The drawing under review shows one solid part. Ordinate dimensions are in mm from its lowest x, y, z. Round coordinates to 2 decimals unless told otherwise and drop trailing zeros. Order: outer loops, then holes, each group sorted by start corner. A loop starts at its lowest first (then second) coordinate and runs counter-clockwise, first axis right, second up. Notation, with made-up numbers: M 72,7.5 L 126,7.5 A17 ccw 126,39.5 Z; hole C 89,84.25 d9. An arc over 180 degrees is marked long. Answer as a JSON object with one key per item and string values. Group by question number.
1) Consider section B-B, the plane x = 72. Write out the cut boundary in (y, z).
2) Insertion check: pin 1 Ø4 at (x, y) = (59.2, 207.89) entering from -Z. The pin has a flat end and moves straight along its axis. Give the tip position at first contact, or say it passes through.
3) Consider section C-C, the plane z = 1.1. Count the separate pieces of the cut face and the enclosed holes in it, then the cut area to 3 significant figures.
4) Consider section A-A, the plane y = 88.5. Write out the cut boundary in (x, z).
5) To check wall thickness, follow line 1 (X direction, y = 257.89, z = 1.65); line 2 (Y direction, x = 138.5, z = 3.4); line 3 (Y direction, x = 173.8, z = 2.5). State the ranges of each line that lie inside material, in increasing order.
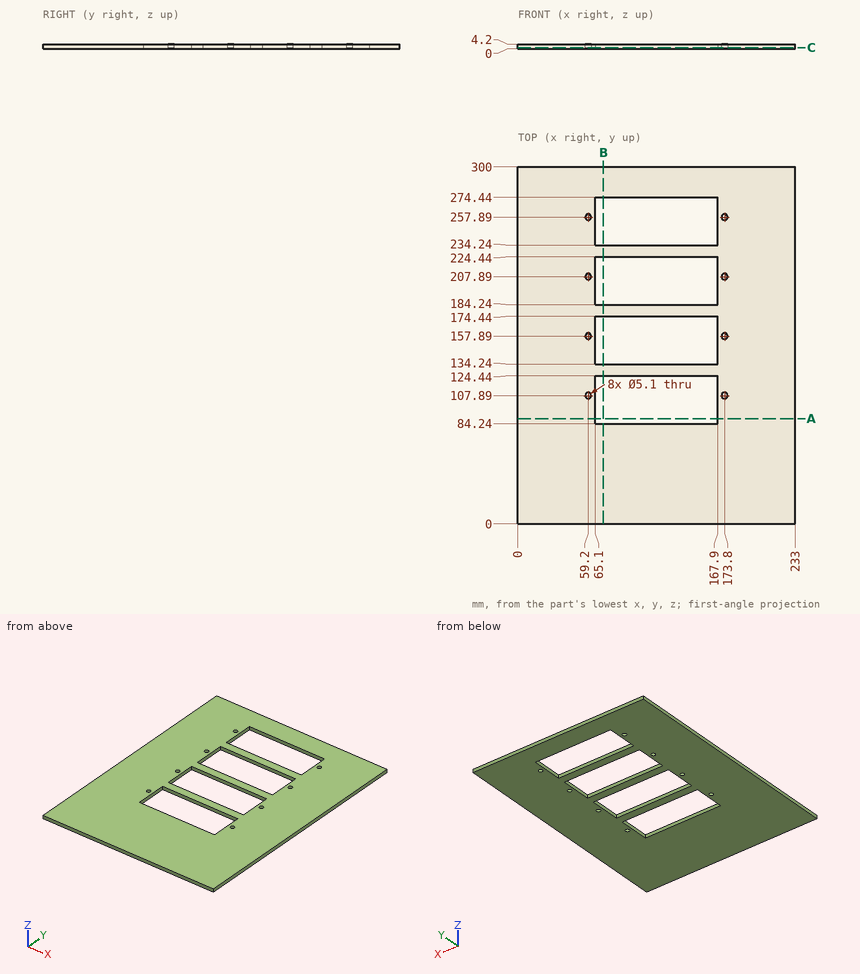
Results list:
{
 "1": {"outline": "M 0,0 L 84.24,0 L 84.24,4.2 L 0,4.2 Z; M 124.44,0 L 134.24,0 L 134.24,4.2 L 124.44,4.2 Z; M 174.44,0 L 184.24,0 L 184.24,4.2 L 174.44,4.2 Z; M 224.44,0 L 234.24,0 L 234.24,4.2 L 224.44,4.2 Z; M 274.44,0 L 300,0 L 300,4.2 L 274.44,4.2 Z"},
 "2": {"pin 1": "through"},
 "3": {"separate pieces": "1", "enclosed holes": "12", "area": "53,200 mm^2"},
 "4": {"outline": "M 0,0 L 65.1,0 L 65.1,4.2 L 0,4.2 Z; M 167.9,0 L 233,0 L 233,4.2 L 167.9,4.2 Z"},
 "5": {"line 1": "0 to 56.65, 61.75 to 65.1, 167.9 to 171.25, 176.35 to 233", "line 2": "0 to 84.24, 124.44 to 134.24, 174.44 to 184.24, 224.44 to 234.24, 274.44 to 300", "line 3": "0 to 105.34, 110.44 to 155.34, 160.44 to 205.34, 210.44 to 255.34, 260.44 to 300"}
}
